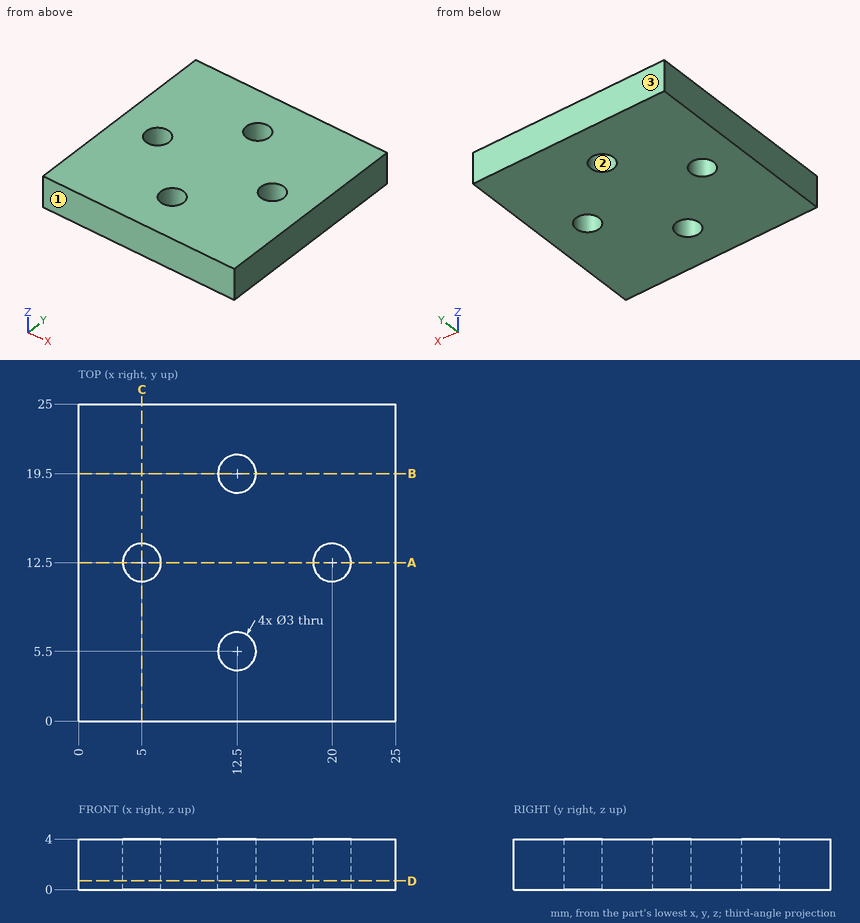
Study the drawing (mm; zero at the part's minimum x, y, z) and answer. Give positions to 0.01 mm unless a question says otherwise; leave off trailing zeros. Write each loop counter-clockwise with the first axis right and the second up, starting at its lowest first coordinate (ties: lowest second). Pieces come first, ordered by that corner, then holes.
(1) The mould has two halves that part along Y. Classify the marked faces 1, 2 and 3: pulls with the +Y half, pulls with the -Y half, needs draft (parallel to the pull), parting line crosses it, or undercut.
Final values:
face 1: pulls with the -Y half
face 2: undercut
face 3: pulls with the +Y half
(2) The part is cut by section B-B on y = 19.5. Write down the section's boundary in (x, z), plus the area to 3 significant figures.
Final values:
outline: (0, 0) - (11, 0) - (11, 4) - (0, 4) - close; (14, 0) - (25, 0) - (25, 4) - (14, 4) - close
area: 88.0 mm2
(3) The part is cut by section A-A on y = 12.5. Write down the section's boundary in (x, z), plus the area to 3 significant figures.
Final values:
outline: (0, 0) - (3.5, 0) - (3.5, 4) - (0, 4) - close; (6.5, 0) - (18.5, 0) - (18.5, 4) - (6.5, 4) - close; (21.5, 0) - (25, 0) - (25, 4) - (21.5, 4) - close
area: 76.0 mm2
(4) Straight lines are drawn through the part: line 1 (X direction, y = 12.5, z = 0.9); line 2 (Y direction, x = 12.5, z = 1.35); line 3 (X direction, y = 5.5, z = 0.85). For each, find the intervals that lie inside material, in ascending order.
Final values:
line 1: x = 0 to 3.5, 6.5 to 18.5, 21.5 to 25
line 2: y = 0 to 4, 7 to 18, 21 to 25
line 3: x = 0 to 11, 14 to 25
(5) The part is cut by section D-D on z = 0.7. Write down the section's boundary in (x, y).
Final values:
outline: (0, 0) - (25, 0) - (25, 25) - (0, 25) - close; hole circle Ø3 at (5, 12.5); hole circle Ø3 at (12.5, 5.5); hole circle Ø3 at (12.5, 19.5); hole circle Ø3 at (20, 12.5)
